from build123d import *
from build123d.topology import SkipClean

# Parameters (mm, degrees)
BOSS_EXTRUDE1_DEPTH     = 11
SHELL1_T                = -1
BOSS_EXTRUDE2_START     = 14
BOSS_EXTRUDE2_DEPTH     = 14
BOSS_EXTRUDE3_START     = 4
BOSS_EXTRUDE3_DEPTH     = 4
CUT_EXTRUDE1_DEPTH      = 73.950753937
CUT_EXTRUDE1_DEPTH_BACK = 73.950753937
SKETCH5_R               = 1.6
CUT_EXTRUDE3_START      = -3
CUT_EXTRUDE3_DEPTH      = 3
SKETCH13_R              = 2.75
BOSS_EXTRUDE4_DEPTH     = 2
SKETCH14_R              = 4
BOSS_EXTRUDE5_DEPTH     = 6
BOSS_EXTRUDE6_START     = -135
BOSS_EXTRUDE6_DEPTH     = 135
BOSS_EXTRUDE7_DEPTH     = 3


with BuildPart() as part:
    # Sketch1 → Boss-Extrude1 (new body)
    with BuildSketch(Plane(origin=(0, 0, 0), x_dir=(1, 0, 0), z_dir=(0, 1, 0))):
        with BuildLine():
            Line((65.5, -23.25), (-65.5, -23.25))
            ThreePointArc((-65.5, -23.25), (-66.914213562, -22.664213562), (-67.5, -21.25))
            Line((-67.5, -21.25), (-67.5, 21.25))
            ThreePointArc((-67.5, 21.25), (-66.914213562, 22.664213562), (-65.5, 23.25))
            Line((-65.5, 23.25), (65.5, 23.25))
            ThreePointArc((65.5, 23.25), (66.914213562, 22.664213562), (67.5, 21.25))
            Line((67.5, 21.25), (67.5, -21.25))
            ThreePointArc((67.5, -21.25), (66.914213562, -22.664213562), (65.5, -23.25))
        make_face()
    extrude(amount=BOSS_EXTRUDE1_DEPTH)

    # Shell1
    shell1_openings = [part.faces().sort_by_distance(p)[0] for p in [
        (0, 0, 0),
    ]]
    offset(amount=SHELL1_T, openings=shell1_openings, kind=Kind.INTERSECTION)

    # Sketch4 → Boss-Extrude2 (add)
    with SkipClean():  # the faces are left unmerged after this step: merging them gives an invalid solid
        with BuildSketch(Plane.XZ.offset(-10).offset(BOSS_EXTRUDE2_START)):
            with BuildLine():
                Line((65.5, -23.25), (60, -23.25))
                Line((60, -23.25), (60, -19.25))
                ThreePointArc((60, -19.25), (61.025126266, -16.775126266), (63.5, -15.75))
                Line((63.5, -15.75), (67.5, -15.75))
                Line((67.5, -15.75), (67.5, -21.25))
                ThreePointArc((67.5, -21.25), (66.914213562, -22.664213562), (65.5, -23.25))
            make_face()
            with BuildLine():
                Line((65.5, 23.25), (60, 23.25))
                Line((60, 23.25), (60, 19.25))
                ThreePointArc((60, 19.25), (61.025126266, 16.775126266), (63.5, 15.75))
                Line((63.5, 15.75), (67.5, 15.75))
                Line((67.5, 15.75), (67.5, 21.25))
                ThreePointArc((67.5, 21.25), (66.914213562, 22.664213562), (65.5, 23.25))
            make_face()
            with BuildLine():
                Line((-67.5, -21.25), (-67.5, -15.75))
                Line((-67.5, -15.75), (-63.5, -15.75))
                ThreePointArc((-63.5, -15.75), (-61.025126266, -16.775126266), (-60, -19.25))
                Line((-60, -19.25), (-60, -23.25))
                Line((-60, -23.25), (-65.5, -23.25))
                ThreePointArc((-65.5, -23.25), (-66.914213562, -22.664213562), (-67.5, -21.25))
            make_face()
            with BuildLine():
                Line((-60, 19.25), (-60, 23.25))
                Line((-60, 23.25), (-65.5, 23.25))
                ThreePointArc((-65.5, 23.25), (-66.914213562, 22.664213562), (-67.5, 21.25))
                Line((-67.5, 21.25), (-67.5, 15.75))
                Line((-67.5, 15.75), (-63.5, 15.75))
                ThreePointArc((-63.5, 15.75), (-61.025126266, 16.775126266), (-60, 19.25))
            make_face()
        extrude(amount=-BOSS_EXTRUDE2_DEPTH)
    add(part.part.scale(1), mode=Mode.REPLACE)  # the faces are merged on a copy

    # Sketch7 → Boss-Extrude3 (add)
    with SkipClean():  # the faces are left unmerged after this step: merging them gives an invalid solid
        with BuildSketch(Plane.XZ.offset(-10).offset(BOSS_EXTRUDE3_START)):
            with BuildLine():
                Line((65.5, -23.25), (60, -23.25))
                Line((60, -23.25), (57, -23.25))
                Line((57, -23.25), (57, -19.633333333))
                Line((57, -19.633333333), (57, -19.25))
                ThreePointArc((57, -19.25), (58.903805922, -14.653805922), (63.5, -12.75))
                Line((63.5, -12.75), (67.5, -12.75))
                Line((67.5, -12.75), (67.5, -15.75))
                Line((67.5, -15.75), (67.5, -21.25))
                ThreePointArc((67.5, -21.25), (66.914213562, -22.664213562), (65.5, -23.25))
            make_face()
            with BuildLine():
                Line((65.5, 23.25), (60, 23.25))
                Line((60, 23.25), (57, 23.25))
                Line((57, 23.25), (57, 19.25))
                ThreePointArc((57, 19.25), (58.903805922, 14.653805922), (63.5, 12.75))
                Line((63.5, 12.75), (67.5, 12.75))
                Line((67.5, 12.75), (67.5, 15.75))
                Line((67.5, 15.75), (67.5, 21.25))
                ThreePointArc((67.5, 21.25), (66.914213562, 22.664213562), (65.5, 23.25))
            make_face()
            with BuildLine():
                Line((-67.5, -21.25), (-67.5, -15.75))
                Line((-67.5, -15.75), (-67.5, -12.75))
                Line((-67.5, -12.75), (-63.5, -12.75))
                ThreePointArc((-63.5, -12.75), (-58.903805922, -14.653805922), (-57, -19.25))
                Line((-57, -19.25), (-57, -23.25))
                Line((-57, -23.25), (-60, -23.25))
                Line((-60, -23.25), (-65.5, -23.25))
                ThreePointArc((-65.5, -23.25), (-66.914213562, -22.664213562), (-67.5, -21.25))
            make_face()
            with BuildLine():
                Line((-67.5, 15.75), (-67.5, 21.25))
                ThreePointArc((-67.5, 21.25), (-66.914213562, 22.664213562), (-65.5, 23.25))
                Line((-65.5, 23.25), (-60, 23.25))
                Line((-60, 23.25), (-57, 23.25))
                Line((-57, 23.25), (-57, 19.25))
                ThreePointArc((-57, 19.25), (-58.903805922, 14.653805922), (-63.5, 12.75))
                Line((-63.5, 12.75), (-67.5, 12.75))
                Line((-67.5, 12.75), (-67.5, 15.75))
            make_face()
        extrude(amount=-BOSS_EXTRUDE3_DEPTH)
    add(part.part.scale(1), mode=Mode.REPLACE)  # the faces are merged on a copy

    # Sketch5 → Cut-Extrude1 (cut, two sides: drawn at the far end of the back side and taken through both)
    with BuildSketch(Plane(origin=(0, 11, 0), x_dir=(1, 0, 0), z_dir=(0, 1, 0)).offset(-CUT_EXTRUDE1_DEPTH_BACK)):
        with Locations(Location((-63.5, 19.25, 0), (0, 0, 270))):
            Circle(SKETCH5_R)
        with Locations(Location((-63.5, -19.25, 0), (0, 0, 270))):
            Circle(SKETCH5_R)
        with Locations(Location((63.5, 19.25, 0), (0, 0, 270))):
            Circle(SKETCH5_R)
        with Locations(Location((63.5, -19.25, 0), (0, 0, 270))):
            Circle(SKETCH5_R)
    extrude(amount=CUT_EXTRUDE1_DEPTH + CUT_EXTRUDE1_DEPTH_BACK, mode=Mode.SUBTRACT)

    # Sketch12 → Cut-Extrude3 (cut)
    with BuildSketch(Plane(origin=(0, 11, 0), x_dir=(1, 0, 0), z_dir=(0, 1, 0)).offset(CUT_EXTRUDE3_START)):
        with BuildLine():
            Line((-63.5, 15.75), (-67.5, 15.75))
            Line((-67.5, 15.75), (-67.5, 21.25))
            ThreePointArc((-67.5, 21.25), (-66.914763627, 22.662885589), (-65.501878037, 23.248121963))
            Line((-65.501878037, 23.248121963), (-60, 23.248121963))
            Line((-60, 23.248121963), (-60, 19.25))
            ThreePointArc((-60, 19.25), (-61.025126266, 16.775126266), (-63.5, 15.75))
        make_face()
        with BuildLine():
            Line((-63.5, -15.75), (-67.5, -15.75))
            Line((-67.5, -15.75), (-67.5, -21.25))
            ThreePointArc((-67.5, -21.25), (-66.914213562, -22.664213562), (-65.5, -23.25))
            Line((-65.5, -23.25), (-60, -23.25))
            Line((-60, -23.25), (-60, -19.25))
            ThreePointArc((-60, -19.25), (-61.025126266, -16.775126266), (-63.5, -15.75))
        make_face()
        with BuildLine():
            Line((60, -19.25), (60, -23.25))
            Line((60, -23.25), (65.5, -23.25))
            ThreePointArc((65.5, -23.25), (66.914213562, -22.664213562), (67.5, -21.25))
            Line((67.5, -21.25), (67.5, -15.75))
            Line((67.5, -15.75), (63.5, -15.75))
            ThreePointArc((63.5, -15.75), (61.025126266, -16.775126266), (60, -19.25))
        make_face()
        with BuildLine():
            Line((60, 19.25), (60, 23.25))
            Line((60, 23.25), (65.5, 23.25))
            ThreePointArc((65.5, 23.25), (66.914213562, 22.664213562), (67.5, 21.25))
            Line((67.5, 21.25), (67.5, 15.75))
            Line((67.5, 15.75), (63.5, 15.75))
            ThreePointArc((63.5, 15.75), (61.025126266, 16.775126266), (60, 19.25))
        make_face()
    extrude(amount=CUT_EXTRUDE3_DEPTH, mode=Mode.SUBTRACT)

    # Sketch13 → Boss-Extrude4 (add)
    with BuildSketch(Plane.XZ.offset(-10)):
        with Locations(Location((-45.5, -7.4, 0), (0, 0, 270))):
            Circle(SKETCH13_R)
    extrude(amount=BOSS_EXTRUDE4_DEPTH)

    # Sketch14 → Boss-Extrude5 (add)
    with BuildSketch(Plane.ZY.offset(67.5)):
        with Locations(Location((4.65, 7, 0), (0, 0, 90))):
            Circle(SKETCH14_R)
    extrude(amount=BOSS_EXTRUDE5_DEPTH)

    # Sketch15 → Boss-Extrude6 (add)
    with BuildSketch(Plane(origin=(67.5, 0, 0), x_dir=(0, 0, -1), z_dir=(1, 0, 0)).offset(BOSS_EXTRUDE6_START)):
        with BuildLine():
            Line((-10, 15), (-10, 11))
            Line((-10, 11), (10, 11))
            Line((10, 11), (10, 15))
            ThreePointArc((10, 15), (0, 13.284271247), (-10, 15))
        make_face()
    extrude(amount=BOSS_EXTRUDE6_DEPTH)

    # Sketch16 → Boss-Extrude7 (add)
    with BuildSketch(Plane.XY.offset(23.25)):
        Polygon((-36, 11), (-32, 11), (-32, 12.5), (-28, 12.5), (-28, 11), (-24, 11), (-24, 14.5), (-36, 14.5), align=None)
        Polygon((24, 11), (28, 11), (28, 12.5), (32, 12.5), (32, 11), (36, 11), (36, 14.5), (24, 14.5), align=None)
    boss_extrude7 = extrude(amount=-BOSS_EXTRUDE7_DEPTH)

    # Mirror1: Boss-Extrude7 across plane
    add(boss_extrude7.mirror(Plane.XY))


solid = part.part
Part model, mm, in its own coordinate system. A direction names the side the tool comes from. Coordinates: 2 decimals unless noted, no trailing zeros. Loops run counter-clockwise (first coordinate to the right, second up) from the corner with the lowest first, then second, coordinate; pieces in that order, holes last. Notation, with made-up numbers: (-11.5, 68.25) - (11.5, 68.25) arc R11 cw to (11.5, 74.25) - close; hole circle Ø11 at (17.25, -25). An arc over 180 degrees is marked (long way). Write each question's results on one line, items separated by ' | '. Start each with the question number.
Q1. Slice it at B-B on z = -1. Give the cut face in (x, y), and give its area (3 significant figures).
Q2. Drop flat-ended pins along their axis: pin 1 Ø5.5 at (y, z) = (10, -3.5) entering from -X; pin 2 Ø0.9 at (y, z) = (9.5, 21) entering from +X; pin 3 Ø2.5 at (x, z) = (-30, -22.5) entering from -Y. Give the stop position or say it passes through.
Q3. Two-plate mould, pull along Z, no slides. Class faces 5 (the flat face through (-36, 13, -22)), 6 (the flat face through (65, 1, -15.75)): +Z half, -Z half, draft (parallel to the pull), parting line (faces both ways), or undercut.
Q4. Slice it at A-A on x = 19. Give the cut face in (y, z), and give its area (3 significant figures).
Q5. Probe line 1 along Z through (x, y) = (-63.5, 2.25); line 2 along X through (y, z) = (1.75, 19.25); line 3 along Z through (x, y) = (-3.5, 9). List the from-to ranges inside material, lowest first.
Q6. Slice it at C-C on z = -7.4. Give the cut face in (x, y).
Q7. Which spindle directions (+Z, -Z, +X, -X, +Y, -Y) get a long thin tool onto all of the face, cutting with end or side? Do faces 1 (the flat face through (-30, 13, 20.25)), 2 (the flat face through (24, 13, -22)), 3 (the flat face through (66.5, 5, 0)), 4 (the flat face through (-64, 8, 21)). Say none if no direction does.
Answer:
1) outline: (-67.5, 0) - (-66.5, 0) - (-66.5, 10) - (66.5, 10) - (66.5, 0) - (67.5, 0) - (67.5, 13.3) - (-67.5, 13.3) - close | area: 466 mm2
2) pin 1: stops at x = -67.5 | pin 2: stops at x = 60 | pin 3: stops at y = 0
3) face 5: draft | face 6: undercut
4) outline: (0, -23.25) - (11, -23.25) - (11, -10) - (15, -10) arc R30 cw to (15, 10) - (11, 10) - (11, 23.25) - (0, 23.25) - (0, 22.25) - (10, 22.25) - (10, -22.25) - (0, -22.25) - close | area: 123 mm2
5) line 1: z = -23.25 to -20.85, -17.65 to -15.75, 15.75 to 17.65, 20.85 to 23.25 | line 2: x = -67.5 to -65.1, -61.9 to -60, 60 to 61.9, 65.1 to 67.5 | line 3: z = -23.25 to -22.25, 22.25 to 23.25
6) outline: (-67.5, 0) - (-66.5, 0) - (-66.5, 10) - (-48.25, 10) - (-48.25, 8) - (-42.75, 8) - (-42.75, 10) - (66.5, 10) - (66.5, 0) - (67.5, 0) - (67.5, 14.21) - (-67.5, 14.21) - close
7) face 1: +X, -X, +Y | face 2: -Z, +Y | face 3: -Y | face 4: +Z, -X, +Y
